Geometry check sheet. Reference: the model listing, model coordinates, mm. Face numbers are marked on the shaded views. Coordinates: 2 decimals unless noted, no trailing zeros. Write each loop counter-clockwise with the first axis right and the second up, starting at its lowest first coordinate (ties: lowest second). Pieces come first, ordered by that corner, then holes. Notation, with made-up numbers: (88, -3.5) -> (94, -3.5) arc R21 ccw to (94, 1.5) -> close; hole circle Ø1 at (79, 13). An arc over 180 degrees is marked (long way). Answer in a Markdown table with one row per item. Add a question column.
1. Depth check by flat-ended pin: P1, Ø1, axis at x = -3, y = -16.5, coming from the -Z side; P2, Ø2, axis at y = -9, z = 2.5, coming from the -X side; P3, Ø3, axis at x = 0, z = 0, coming from the +Y side; P4, Ø3, axis at x = -1, z = 0, coming from the +Y side. Enter the tip coordinate at first touch or a pass-through.
2. Cross-section at B-B on x = 0. Record the cut outline in (y, z), and give its area (3 significant figures).
3. Cross-section at A-A on z = 0. Record the cut outline in (x, y), and give its area (3 significant figures).
4. Mould release check, pull along Z, two halves, no side actions. Record for the marked faces 1, 2 and 3: pulls with the +Z half, pulls with the -Z half, needs draft (parallel to the pull), parting line crosses it, or undercut.
5. Cross-section at D-D on y = -6. Record the cut outline in (x, z).
6. Scan lines: L1, parallel to Z at x = 0, y = -4.5; L2, parallel to Y at x = -3.5, z = 1.5. Record each from-to range of solid material in increasing order. Write a range as from..to.
7. Cross-section at C-C on y = -37.5. Record the cut outline in (x, z), and give its area (3 significant figures).
```python
from build123d import *

# Parameters (mm, degrees)
ESQUISSE1_R             = 4
BOSS_EXTRU_1_DEPTH      = 39
ESQUISSE3_R             = 2
ENL_V_MAT_EXTRU_1_DEPTH = 10
ESQUISSE4_R             = 2
BOSS_EXTRU_2_DEPTH      = 5


with BuildPart() as part:
    # Esquisse1 → Boss.-Extru.1 (new body)
    with BuildSketch(Plane(origin=(0, 0, 0), x_dir=(1, 0, 0), z_dir=(0, 1, 0))):
        Circle(ESQUISSE1_R)
    extrude(amount=-BOSS_EXTRU_1_DEPTH)

    # Esquisse3 → Enlèv. mat.-Extru.1 (cut)
    with BuildSketch(Plane(origin=(0, 0, 0), x_dir=(1, 0, 0), z_dir=(0, 1, 0))):
        Circle(ESQUISSE3_R)
    extrude(amount=-ENL_V_MAT_EXTRU_1_DEPTH, mode=Mode.SUBTRACT)

    # Esquisse4 → Boss.-Extru.2 (add)
    with BuildSketch(Plane.XZ.offset(39)):
        Circle(ESQUISSE4_R)
    extrude(amount=BOSS_EXTRU_2_DEPTH)


solid = part.part
```
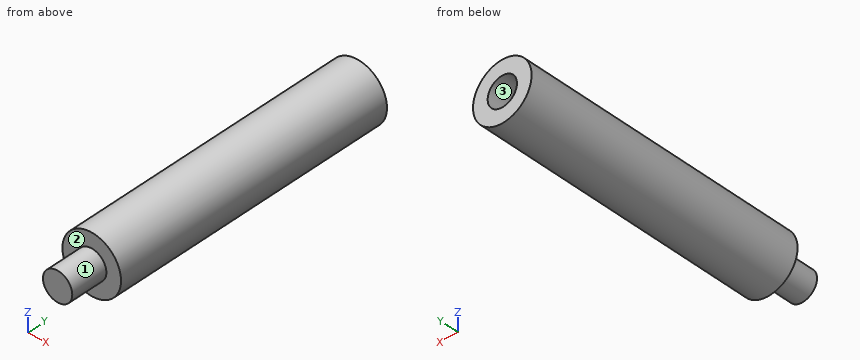
Results found:
| question | item | result |
|---|---|---|
| 1 | P1 | stops at z = -3.12 |
| 1 | P2 | stops at x = -3.71 |
| 1 | P3 | stops at y = -10 |
| 1 | P4 | stops at y = 0 |
| 2 | outline | (-44, -2) -> (-39, -2) -> (-39, -4) -> (0, -4) -> (0, -2) -> (-10, -2) -> (-10, 2) -> (0, 2) -> (0, 4) -> (-39, 4) -> (-39, 2) -> (-44, 2) -> close |
| 2 | area | 292 mm^2 |
| 3 | outline | (-4, -39) -> (-2, -39) -> (-2, -44) -> (2, -44) -> (2, -39) -> (4, -39) -> (4, 0) -> (2, 0) -> (2, -10) -> (-2, -10) -> (-2, 0) -> (-4, 0) -> close |
| 3 | area | 292 mm^2 |
| 4 | face 1 | parting line crosses it |
| 4 | face 2 | needs draft |
| 4 | face 3 | undercut |
| 5 | outline | circle Ø8 at (0, 0); hole circle Ø4 at (0, 0) |
| 6 | L1 | z = -4..-2, 2..4 |
| 6 | L2 | y = -39..0 |
| 7 | outline | circle Ø8 at (0, 0) |
| 7 | area | 50.3 mm^2 |
